Job drawing, mm, ordinate dimensions from the low corner. One solid piece. A direction names the side the tool comes from. Give positions to 0.01 mm unless a question says otherwise; leave off trailing zeros. Loops run counter-clockwise (first coordinate to the right, second up) from the corner with the lowest first, then second, coordinate; pieces in that order, holes last. Notation, with made-up numbers: M -12.75,-38.75 L 45.25,-38.75 A26 cw 45.25,-5.75 Z; hole C -2,-12.5 d8. An arc over 180 degrees is marked long. Answer in a Markdown table with one row per item.
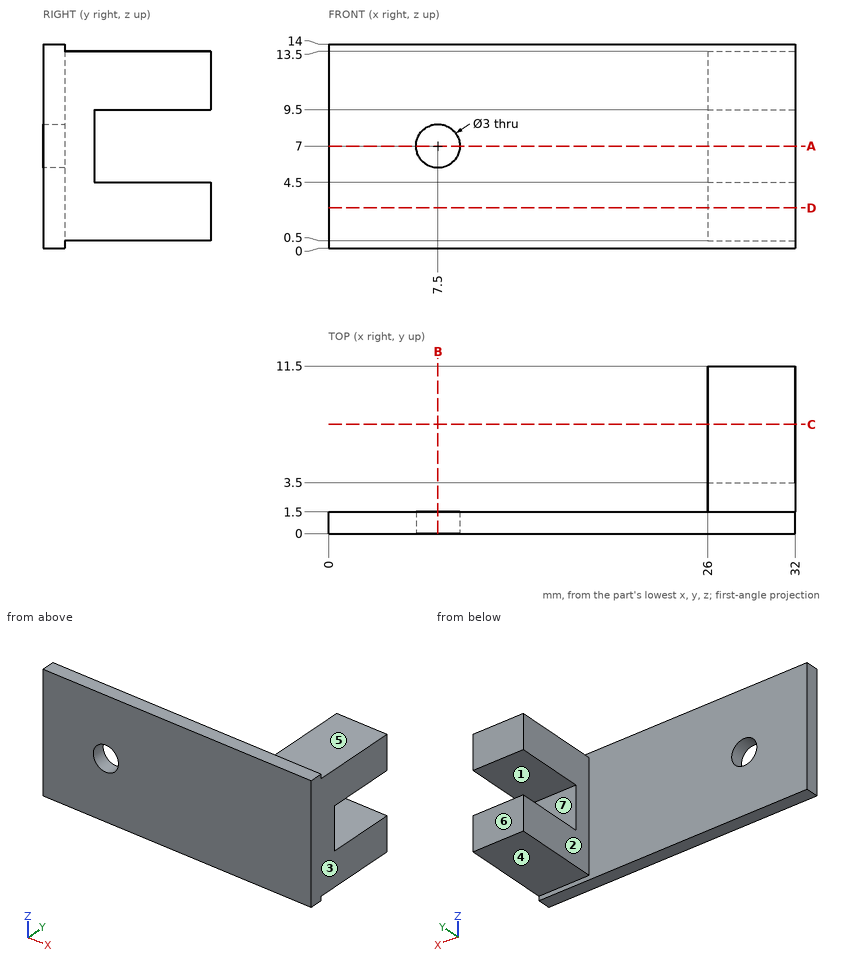
(1) Saw through at D-D (z = 2.75). Write the cut outline in (x, y), plus the area to 3 significant figures.
Recorded:
| item | result |
|---|---|
| outline | M 0,0 L 32,0 L 32,11.5 L 26,11.5 L 26,1.5 L 0,1.5 Z |
| area | 108 mm^2 |
(2) Pull direction Z, two halves, no side cores. Call the marked faces 4, 5, 6 and 7: +Z half, -Z half, draft (parallel to the pull), parting line (faces both ways), or undercut.
Recorded:
| item | result |
|---|---|
| face 4 | -Z half |
| face 5 | +Z half |
| face 6 | draft |
| face 7 | undercut |
(3) Saw through at A-A (z = 7). Write the cut outline in (x, y), plus the area to 3 significant figures.
Recorded:
| item | result |
|---|---|
| outline | M 0,0 L 6,0 L 6,1.5 L 0,1.5 Z; M 9,0 L 32,0 L 32,3.5 L 26,3.5 L 26,1.5 L 9,1.5 Z |
| area | 55.5 mm^2 |
(4) Saw through at C-C (y = 7.5). Write the cut outline in (x, z), plus the area to 3 significant figures.
Recorded:
| item | result |
|---|---|
| outline | M 26,0.5 L 32,0.5 L 32,4.5 L 26,4.5 Z; M 26,9.5 L 32,9.5 L 32,13.5 L 26,13.5 Z |
| area | 48.0 mm^2 |
(5) Drill centre lines: line 1 along Z through (x, y) = (29, 5.5); line 2 along Y through (x, z) = (18, 12); line 3 along X through (y, z) = (1.05, 7). Where is each one in solid material? Low to high.
Recorded:
| item | result |
|---|---|
| line 1 | z = 0.5 to 4.5, 9.5 to 13.5 |
| line 2 | y = 0 to 1.5 |
| line 3 | x = 0 to 6, 9 to 32 |
(6) Pin check, flat tips, straight feed: pin 1 Ø6.5 at (x, y) = (28.5, 7.5) entering from -Z; pin 2 Ø1.5 at (x, y) = (28, 7) entering from +Z; pin 3 Ø1.5 at (x, z) = (15, 6.5) entering from +Y. Stop position of each tip, or through.
Recorded:
| item | result |
|---|---|
| pin 1 | stops at z = 0.5 |
| pin 2 | stops at z = 13.5 |
| pin 3 | stops at y = 1.5 |
(7) Which spindle directions (+Z, -Z, +X, -X, +Y, -Y) get a long thin tool onto all of the face, cutting with end or side? Do the marked faces 1, 2 and 3. Say none if no direction does.
Recorded:
| item | result |
|---|---|
| face 1 | +X, -X, +Y |
| face 2 | +Z, -Z, -X, +Y |
| face 3 | +Z, -Z, +X, +Y, -Y |
(8) Saw through at B-B (x = 7.5). Write the cut outline in (y, z), plus the area to 3 significant figures.
Recorded:
| item | result |
|---|---|
| outline | M 0,0 L 1.5,0 L 1.5,5.5 L 0,5.5 Z; M 0,8.5 L 1.5,8.5 L 1.5,14 L 0,14 Z |
| area | 16.5 mm^2 |
